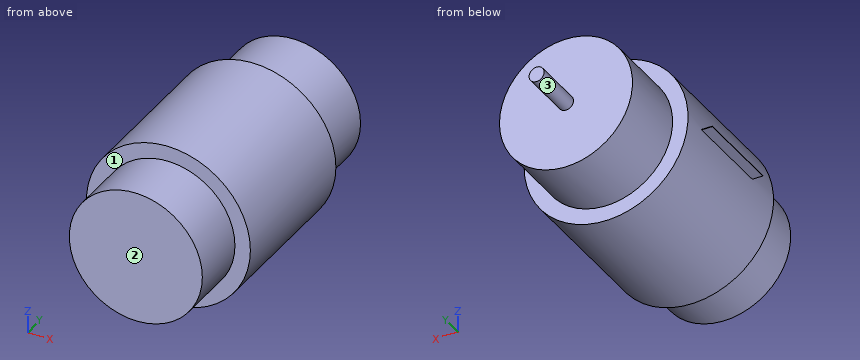
```python
from build123d import *

# Parameters (mm, degrees)
F0_R     = 14
F1_DEPTH = 59.2
F3_START = 15
F2_R     = 17.25
F3_DEPTH = 32
F4_R     = 1.585
F5_DEPTH = 11
F6_W     = 4.3914923444
F6_H     = 18.9632624388
F7_DEPTH = 0.1


with BuildPart() as f1:
    # F0 (on Front) → F1 (new body)
    with BuildSketch(Plane.XZ):
        Circle(F0_R)
    extrude(amount=F1_DEPTH)

    # F2 (on Front) → F3 (join)
    with BuildSketch(Plane.XZ.offset(F3_START)):
        Circle(F2_R)
    extrude(amount=F3_DEPTH)

    # F4 (on Front) → F5 (join)
    with BuildSketch(Plane.XZ):
        Circle(F4_R)
    extrude(amount=-F5_DEPTH)

    # F6 (on Top) → F7 (join)
    with BuildSketch(Plane.XY):
        with Locations((-17.2895635478, -29.550164938)):
            Rectangle(F6_W, F6_H)
    extrude(amount=F7_DEPTH)


solid = f1.part
```
Geometry check sheet. Reference: the model listing, model coordinates, mm. Face numbers are marked on the shaded views. A direction names the side the tool comes from. Coordinates: 2 decimals unless noted, no trailing zeros. Loops run counter-clockwise (first coordinate to the right, second up) from the corner with the lowest first, then second, coordinate; pieces in that order, holes last.
Item 1: Sectioned sample at A-A, the plane z = 10. Record the boundary of the cut face in (x, y).
Item 2: Sectioned sample at B-B, the plane x = 0. Record the boundary of the cut face in (y, z) (3 decimals), then the cut area to 3 significant figures.
Item 3: Sectioned sample at C-C, the plane y = -24. Record the boundary of the cut face in (x, z), then the cut area to 3 significant figures.
Item 4: Sectioned sample at D-D, the plane z = 6.5. Record the boundary of the cut face in (x, y), then the cut area to 3 significant figures.
Item 5: Thickness scan on line 1 (Y direction, x = 14.5, z = -2.5); line 2 (Y direction, x = 12, z = -0.5); line 3 (Z direction, x = 5.5, y = -42). Record the ranges inside material, lowest first.
Item 6: Go/stop test with flat-tipped pins: pin 1 Ø8 at (x, y) = (-12.5, -37.5) entering from -Z; pin 2 Ø8 at (x, y) = (-11.5, -26.5) entering from -Z; pin 3 Ø8 at (x, y) = (-3.5, -26.5) entering from -Z; pin 4 Ø1.1 at (x, y) = (-18.5, -28) entering from -Z. Record where each tip stops, or that it passes through.
Item 7: Access from +Z, -Z, +X, -X, +Y, -Y to the whole of each face (thin tool, end or side, straight path). Record for the marked faces 1, 2 and 3.
Check result:
1. outline: (-14.06, -47) - (-9.8, -47) - (-9.8, -59.2) - (9.8, -59.2) - (9.8, -47) - (14.06, -47) - (14.06, -15) - (9.8, -15) - (9.8, 0) - (-9.8, 0) - (-9.8, -15) - (-14.06, -15) - close
2. outline: (-59.2, -14) - (-47, -14) - (-47, -17.25) - (-15, -17.25) - (-15, -14) - (0, -14) - (0, -1.585) - (11, -1.585) - (11, 1.585) - (0, 1.585) - (0, 14) - (-15, 14) - (-15, 17.25) - (-47, 17.25) - (-47, 14) - (-59.2, 14) - close
2. area: 1,900 mm2
3. outline: (-19.49, 0) - (-17.25, 0) arc R17.25 ccw (long way) to (-17.25, 0.1) - (-19.49, 0.1) - close
3. area: 935 mm2
4. outline: (-15.98, -47) - (-12.4, -47) - (-12.4, -59.2) - (12.4, -59.2) - (12.4, -47) - (15.98, -47) - (15.98, -15) - (12.4, -15) - (12.4, 0) - (-12.4, 0) - (-12.4, -15) - (-15.98, -15) - close
4. area: 1,700 mm2
5. line 1: y = -47 to -15
5. line 2: y = -59.2 to 0
5. line 3: z = -16.35 to 16.35
6. pin 1: stops at z = -15.01
6. pin 2: stops at z = -15.53
6. pin 3: stops at z = -17.25
6. pin 4: stops at z = 0
7. face 1: -Y
7. face 2: +Z, -Z, +X, -X, -Y
7. face 3: +Y
